Input: part model. Units: mm. Frame: model coordinates. A direction names the side the tool comes from. Coordinates: 2 decimals unless noted, no trailing zeros. Loops run counter-clockwise (first coordinate to the right, second up) from the corner with the lowest first, then second, coordinate; pieces in that order, holes last. Notation, with made-up numbers: (5.5, 38.25) - (28.5, 38.25) arc R24 cw to (28.5, 54.25) - close; hole circle Ø3 at (63, 5.5). An arc over 180 degrees is marked (long way). Use one line per item in the form item = value.
from build123d import *

# Parameters (mm, degrees)
F1_DEPTH = 152.4
F2_R     = 1.98374
F3_R     = 3.69316
F4_R     = 4.7625
F5_R     = 2.38125
F6_DEPTH = 22.225


with BuildPart() as f1:
    # F0 (on Top) → F1 (new body)
    with BuildSketch(Plane.XY):
        Polygon((0, 11.50874), (0, 0), (-18.80616, 0), (-18.80616, 11.50874), (-20.51558, 11.50874), (-20.51558, -1.70942), (1.70942, -1.70942), (1.70942, 11.50874), align=None)
    extrude(amount=F1_DEPTH)

    # F2
    f2_edges = [f1.edges().sort_by_distance(p)[0] for p in [
        (0, 0, 76.2),
        (-18.80616, 0, 76.2),
    ]]
    fillet(f2_edges, radius=F2_R)

    # F3
    f3_edges = [f1.edges().sort_by_distance(p)[0] for p in [
        (1.70942, -1.70942, 76.2),
        (-20.51558, -1.70942, 76.2),
    ]]
    fillet(f3_edges, radius=F3_R)

    # F4
    f4_edges = [f1.edges().sort_by_distance(p)[0] for p in [
        (0.85471, 11.50874, 152.4),
        (-19.66087, 11.50874, 152.4),
        (-19.66087, 11.50874, 0),
        (0.85471, 11.50874, 0),
    ]]
    fillet(f4_edges, radius=F4_R)

    # F5 (on face) → F6 (cut, through all)
    with BuildSketch(Plane.YZ.offset(1.70942)):
        with Locations((6.74624, 4.7625)):
            Circle(F5_R)
        with Locations((6.74624, 147.6375)):
            Circle(F5_R)
    extrude(amount=-F6_DEPTH, mode=Mode.SUBTRACT)


solid = f1.part
Q1. Cut plane B-B, the plane x = -6.25. Return loops of the section in (y, z), then the cut area to 3 significant figures.
Check values:
outline = (-1.71, 0) - (0, 0) - (0, 152.4) - (-1.71, 152.4) - close
area = 261 mm²
Q2. Cut plane A-A, the plane z = 99. Return loops of the section in (x, y).
Check values:
outline = (-20.52, 1.98) arc R3.69 ccw to (-16.82, -1.71) - (-1.98, -1.71) arc R3.69 ccw to (1.71, 1.98) - (1.71, 11.51) - (0, 11.51) - (0, 1.98) arc R1.98 cw to (-1.98, 0) - (-16.82, 0) arc R1.98 cw to (-18.81, 1.98) - (-18.81, 11.51) - (-20.52, 11.51) - close
Q3. First-contact query: P1, Ø4.5, axis at y = 6.75, z = 147.64, coming from the +X side; P2, Ø1.5, axis at x = -8, z = 61, coming from the +Y side. Flat tips, straight axial feed; report the tip coordinate or a pass-through.
Check values:
P1 = through
P2 = 0
Q4. Ray query, line 1 along X through (y, z) = (3, 29); line 2 along Y through (x, z) = (-13.5, 67.5); line 3 along X through (y, z) = (1, 22). Return the intervals inside material, ascending. Write a range as [from, to].
Check values:
line_1 = [-20.52, -18.81], [0, 1.71]
line_2 = [-1.71, 0]
line_3 = [-20.38, -18.55], [-0.26, 1.58]
Q5. Pull-direction query (Z, two-part tool) for faces 1 (the flat face through (-9, 0, 75)), 2 (the cylindrical face through (-19.649, 6.23, 145.313)), 3 (the flat face through (-9.6, -0.2, 0)), 4 (the cylindrical face through (0.867, 7.845, 2.65)); classes: pulls with the +Z half, pulls with the -Z half, needs draft (parallel to the pull), parting line crosses it, or undercut.
Check values:
face_1 = needs draft
face_2 = undercut
face_3 = pulls with the -Z half
face_4 = undercut
Q6. Set-up query: faces 5 (the cylindrical face through (-19, -1, 77)), 6 (the flat face through (-18.806, 7, 75)). Return all of +Z, -Z, +X, -X, +Y, -Y with unobstructed straight access to the full face (end or side cutting, diameter ignored); none if empty.
Check values:
face_5 = +Z, -Z, -X, -Y
face_6 = +Z, -Z, +Y
